Can you work these out from the model? Positions are in its coordinate system, mm. Face numbers are marked on the shaded views. A direction names the side the tool comes from. Give positions to 0.01 mm unless a question says otherwise; leave off trailing zeros. Order: outer loops, then holes, each group sorted by start corner. A loop starts at its lowest first (then second) coordinate and runs counter-clockwise, first axis right, second up. Notation, with made-up numbers: (82.5, 36) -> (88.5, 36) arc R9 cw to (88.5, 48) -> close; hole circle Ø6 at (-20, -22.5). An arc over 180 degrees is marked (long way). Answer as CSV lines item,"result".
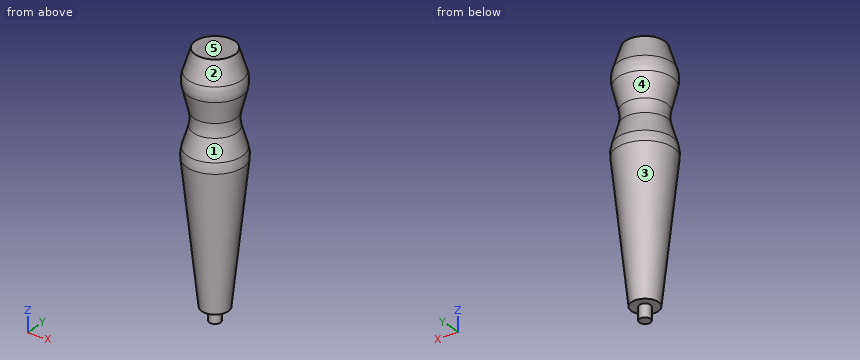
```python
from build123d import *

# Parameters (mm, degrees)
F2_R = 10


with BuildPart() as f1:
    # F0 (on Front) → F1 (revolve)
    with BuildSketch(Plane.XZ):
        Polygon((-11, 55), (-5.1, 0), (-2.1, 0), (-2.1, -5), (0, -5), (0, 92), (-7.5, 92), (-11, 81), (-7.5, 67), align=None)
    revolve(axis=Axis((0, 0, 43.5), (0, 0, -1)))

    # F2
    f2_edges = [f1.edges().sort_by_distance(p)[0] for p in [
        (11, 0, 55),
        (7.5, 0, 67),
        (11, 0, 81),
    ]]
    fillet(f2_edges, radius=F2_R)


solid = f1.part
```
Item 1: Please list where these lines run through material, in increasing order: line 1 along Z through (x, y) = (4.25, 2.75); line 2 along X through (y, z) = (-4.75, 4.5); line 3 along Y through (x, z) = (-6, 75).
Numbers:
line 1,"z = 0 to 92"
line 2,"x = -2.93 to 2.93"
line 3,"y = -7.37 to 7.37"
Item 2: For pin 1 (1 mm diameter, centred on x = -3, y = -0.5, fed in from -Z); pin 2 (12 mm diameter, centred on x = 5.5, z = 60, fed in from -Y); pin 3 (1 mm diameter, centred on y = 2, z = 66.5, fed in from +X), each with a flat end and sliding along its axis, tell me the tip position at first contact or that it passes through.
Numbers:
pin 1,"stops at z = 0"
pin 2,"stops at y = -10.64"
pin 3,"stops at x = 7.75"
Item 3: Imagine slicing it at B-B, the plane z = 34.5. Please give me the cut outline in (x, y), then the cut area to 3 significant figures.
Numbers:
outline,"circle Ø17.6 at (0, 0)"
area,"243 mm²"
Item 4: For the marked faces 1 and 2, which set-ups out of +Z, -Z, +X, -X, +Y, -Y let a thin tool reach every point of the face, with its end or its side?
Numbers:
face 1,"none"
face 2,"+Z"
Item 5: Imagine slicing it at A-A, the plane z = 59.5. Please give me the cut outline in (x, y) (1 decimal), then the cut area to 3 significant figures.
Numbers:
outline,"circle Ø19.4 at (0, 0)"
area,"295 mm²"
Item 6: We'd pull the mould along Z, two halves only. Please class the marked faces 3, 4 and 5: released by +Z, released by -Z, zero draft, split by the parting line, or undercut.
Numbers:
face 3,"released by -Z"
face 4,"undercut"
face 5,"released by +Z"
